For this review, take the finished solid that the model builds, in its own axes (mm). Give positions to 0.01 mm unless a question says otherwise; leave off trailing zeros. Loops run counter-clockwise (first coordinate to the right, second up) from the corner with the lowest first, then second, coordinate; pieces in that order, holes last. Notation, with made-up numbers: (34, 17) - (41, 17) arc R31 cw to (41, 44) - close; hole circle Ø6 at (40.25, -6). An arc over 180 degrees is marked (long way). Put each result on its own line as item: value.
from build123d import *

# Parameters (mm, degrees)
F0_R        = 30
F0_R_2      = 27.5
F3_R        = 30
F3_R_2      = 27.5
F4_DEPTH    = 30
F2_FACE_R   = 30
F2_FACE_R_2 = 27.5
F5_DEPTH    = 30


with BuildPart() as f2:
    # F2: sweep along a path in F1
    with BuildLine(Plane.XZ) as f2_path:
        ThreePointArc((75, 75), (21.966991, 53.033009), (0, 0))
    # F0 (on Top) → F2 (sweep)
    with BuildSketch(Plane.XY):
        Circle(F0_R)
        Circle(F0_R_2, mode=Mode.SUBTRACT)
    sweep(path=f2_path.line)

    # F3 (on face) → F4 (join)
    with BuildSketch(Plane.YZ.offset(75)):
        with Locations((0, 75)):
            Circle(F3_R)
        with Locations((0, 75)):
            Circle(F3_R_2, mode=Mode.SUBTRACT)
    extrude(amount=F4_DEPTH)

    # F2_face (on face) → F5 (join)
    with BuildSketch(Plane(origin=(0, 0, 0), x_dir=(1, 0, 0), z_dir=(0, 0, -1))):
        Circle(F2_FACE_R)
        Circle(F2_FACE_R_2, mode=Mode.SUBTRACT)
    extrude(amount=F5_DEPTH)


solid = f2.part
1) Take a section at A-A on y = 0. State the section outline as (x, z) points, and give its area (3 significant figures).
Geometry check:
outline: (-30, -30) - (-27.5, -30) - (-27.5, 0) arc R102.5 cw to (75, 102.5) - (105, 102.5) - (105, 105) - (75, 105) arc R105 ccw to (-30, 0) - close; (27.5, -30) - (30, -30) - (30, 0) arc R45 cw to (75, 45) - (105, 45) - (105, 47.5) - (75, 47.5) arc R47.5 ccw to (27.5, 0) - close
area: 889 mm²
2) Take a section at B-B on z = -17. State the section outline as (x, y) points, and give its area (3 significant figures).
Geometry check:
outline: circle Ø60 at (0, 0); hole circle Ø55 at (0, 0)
area: 452 mm²
3) Take a section at C-C on y = 9.5. State the section outline as (x, z) points.
Geometry check:
outline: (-28.46, -30) - (-25.81, -30) - (-25.81, 0) arc R100.81 cw to (75, 100.81) - (105, 100.81) - (105, 103.46) - (75, 103.46) arc R103.46 ccw to (-28.46, 0) - close; (25.81, -30) - (28.46, -30) - (28.46, 0) arc R46.54 cw to (75, 46.54) - (105, 46.54) - (105, 49.19) - (75, 49.19) arc R49.19 ccw to (25.81, 0) - close
4) Insertion check: pin 1 Ø1 at (y, z) = (-13.5, 2) entering from -X; pin 2 Ø2 at (x, y) = (-13, 6.5) entering from -Z; pin 3 Ø4 at (y, z) = (0, 33.5) entering from +X. Each pin has a flat end and moves straight along its axis. Give the tip position at first contact, or say it passes through.
Geometry check:
pin 1: stops at x = -27.02
pin 2: stops at z = 49.18
pin 3: stops at x = 47.35
5) Wall thickness on line 1 (Y direction, x = 99, z = 75); line 2 (Z direction, x = 95, y = 0): over which ranges is each line inside the solid? List them lowest first.
Geometry check:
line 1: y = -30 to -27.5, 27.5 to 30
line 2: z = 45 to 47.5, 102.5 to 105
6) Draft analysis for pull direction X (two halves, no side actions). For faces 1 (the face through (-5.961, 26.846, -14.79)), 2 (the face through (105, 24.3, 61.8)), 3 (the face through (13.2, 24.3, -30)), 4 (the face through (27.712, 11.49, -14.79)), state which applies: pulls with the +X half, pulls with the -X half, needs draft (parallel to the pull), parting line crosses it, or undercut.
Geometry check:
face 1: undercut
face 2: pulls with the +X half
face 3: needs draft
face 4: parting line crosses it
